Autodesk Inventor part; units mm, degrees
ref_plane "XZ Plane" through (0, 0, 0) normal (0, 1, 0) x (-1, 0, 0)
ref_plane "XY Plane" through (0, 0, 0) normal (0, 0, 1) x (1, 0, 0)
sketch "Sketch1" plane through (0, 0, 0) normal (0, 0, 1) x (1, 0, 0)
  line L0 (125.1975, -635.9781) -> (-63.4844, -635.9781)
  line L1 (-63.4844, -635.9781) -> (-63.4844, -848.7632)
  line L2 (-63.4844, -848.7632) -> (125.1975, -848.7632)
  line L3 (125.1975, -848.7632) -> (125.1975, -635.9781)
  point P0 (0, 0)
extrude "Extrusion1" add sketch "Sketch1" along normal blind 144.4625
sketch "Sketch2" plane through (-63.4844, -848.7632, 0) normal (0, -1, 0) x (1, 0, 0)
  line L0 (188.6819, 144.4625) -> (0, 144.4625)
  line L1 (0, 0) -> (0, 144.4625)
  line L2 (188.6819, 0) -> (188.6819, 144.4625)
  line L3 (0, 17.8487) -> (30.8457, 144.4625)
  line L4 (30.8457, 144.4625) -> (188.6819, 109.8581)
  point P0 (63.4844, 0)
extrude "Extrusion2" cut sketch "Sketch2" against normal through all
sketch "Sketch3" plane through (-63.4844, -848.7632, 17.8487) normal (-0.9715834, 0, 0.2366975) x (0.2366975, 0, 0.9715834)
  line L0 (0, 0) -> (0, 212.7851)
  circle A0 centre (61.7012, 50.3399) radius 23.1304
  line L1 (15.4405, 202.9114) -> (25.6712, 202.9114)
  line L2 (25.6712, 202.9114) -> (25.6712, 176.2225)
  line L3 (25.6712, 176.2225) -> (15.4405, 176.2225)
  line L4 (15.4405, 176.2225) -> (15.4405, 202.9114)
  line L5 (15.4405, 172.4314) -> (25.6712, 172.4314)
  line L6 (25.6712, 172.4314) -> (25.6712, 145.7425)
  line L7 (25.6712, 145.7425) -> (15.4405, 145.7425)
  line L8 (15.4405, 145.7425) -> (15.4405, 172.4314)
  line L9 (15.4405, 141.9514) -> (25.6712, 141.9514)
  line L10 (25.6712, 141.9514) -> (25.6712, 115.2625)
  line L11 (25.6712, 115.2625) -> (15.4405, 115.2625)
  line L12 (15.4405, 115.2625) -> (15.4405, 141.9514)
  point P0 (-2.3149, 848.7632)
  dimension "d6" = 30.48
extrude "Extrusion3" add sketch "Sketch3" along normal blind 12.7
sketch "Sketch4" plane through (-61.219, -798.4232, 80.8026) normal (-0.9715834, 0, 0.2366975) x (0.2366975, 0, 0.9715834)
  circle A0 centre (0, 0) radius 23.1304
  point P0 (-64.0161, 798.4232)
extrude "Extrusion4" add sketch "Sketch4" along normal blind 12.7
sketch "Sketch5" plane through (-63.4844, -848.7632, 17.8487) normal (-0.9715834, 0, 0.2366975) x (0.2366975, 0, 0.9715834)
  circle A0 centre (61.7012, 50.3399) radius 23.1304
  circle A1 centre (61.7012, 50.3399) radius 29.0734 construction
  circle A2 centre (61.7012, 50.3399) radius 43.7714 construction
  line L0 (61.7012, 50.3399) -> (82.0253, 11.5731) construction
  arc A3 (94.4221, 21.2663) -> (38.4943, 67.8529) centre (67.5786, 45.9046) ccw
  line L1 (75.2007, 24.5906) -> (94.4221, 21.2663)
  arc A4 (75.2007, 24.5906) -> (38.4943, 67.8529) centre (61.7012, 50.3399) ccw
  point P0 (-2.3149, 848.7632)
  dimension "d15" = 87.5428
  dimension "d16" = 58.1469
extrude "Extrusion5" cut sketch "Sketch5" along normal mid plane 12.7 contours L1 A4 A3
fillet "Fillet1" radius 130.175 1 edges at (125.1975, -742.3706, 109.8581)
fillet "Fillet2" radius 4.7625 1 edges at (-79.033, -798.4232, 61.3356)
chamfer "Chamfer1" distance 14.2875 angle 45 1 edges at (-32.6387, -742.3706, 144.4625)
ref_plane "Work Plane1" through (119.0625, 0, 0) normal (1, 0, 0) x (0, 1, 0)
sketch "Sketch6" plane through (119.0625, 0, 0) normal (1, 0, 0) x (0, 1, 0)
  circle A0 centre (-684.0193, 29.4352) radius 9.6445
  point P0 (0, 0)
extrude "Extrusion6" add sketch "Sketch6" along normal blind 12.7
properties part number "VoltageSource"
Read the model definition and answer for the solid it produces. Units are mm, in the model's axes. A direction names the side the tool comes from. Give positions to 0.01 mm unless a question says otherwise; leave off trailing zeros. Write each loop counter-clockwise with the first axis right and the second up, starting at its lowest first coordinate (ties: lowest second). Pieces come first, ordered by that corner, then holes. Notation, with made-up numbers: (16, 56) -> (71, 56) arc R20 ccw to (71, 91) -> close; hole circle Ø5 at (9.25, 11.5). An arc over 180 degrees is marked (long way). Answer as a JSON object with one key per item and string values.
1) Straight lines are drawn through the part: probe 1 along X at (y, z) = (-649.5, 49.5); probe 2 along X at (y, z) = (-709.5, 80); probe 3 along Y at (x, z) = (-49.5, 94.5). For each, find the intervals that lie inside material, in ascending order. Write a range as from..to.
Findings below:
{"probe 1": "x = -55.77..117.4", "probe 2": "x = -48.34..101.51", "probe 3": "y = -815.05..-781.8"}
2) Section D-D on x = 62.5 is taken. Write down the section's boundary in (y, z), then the cut area to 3 significant figures.
Findings below:
{"outline": "(-848.76, 0) -> (-635.98, 0) -> (-635.98, 116.45) -> (-848.76, 116.45) -> close", "area": "24,800 mm^2"}
3) A tool of negligible diameter and unlimited length cuts with its end or side. For faces 1 (the flat face through (-65, -706.812, 39)), 2 (the flat face through (-65, -645.852, 39)), 3 (the flat face through (-65.91, -659.38, 34.33)), from which of +Z, -Z, +X, -X, +Y, -Y can it reach the whole face along a straight path? Write none if from no direction.
Findings below:
{"face 1": "+Z, -X", "face 2": "+Z, -X, +Y", "face 3": "-X, +Y, -Y"}
4) For a pull along Y with two mould halves and no side action, classify faces 4 (the flat face through (-63.491, -719.969, 44.272)), 5 (the flat face through (-65, -733.501, 39)), 6 (the flat face through (-65, -676.332, 39)), 7 (the cylindrical face through (127.38, -686.11, 38.85)) as pulls with the +Y half, pulls with the -Y half, needs draft (parallel to the pull), parting line crosses it, or undercut.
Findings below:
{"face 4": "needs draft", "face 5": "pulls with the -Y half", "face 6": "undercut", "face 7": "parting line crosses it"}
5) Section B-B on z = 9 is taken. Write down the section's boundary in (x, y).
Findings below:
{"outline": "(-63.48, -848.76) -> (125.14, -848.76) -> (125.14, -635.98) -> (-63.48, -635.98) -> close"}
6) Flat-ended cylindrical pins translate along their axes: pin 1 Ø4 at (x, z) = (-65.5, 40.5) entering from -Y; pin 2 Ø1 at (y, z) = (-693.5, 117) entering from -X; pin 3 Ø14 at (x, z) = (-68, 39) entering from +Y. Find the tip coordinate at first contact, or state that the pin passes through.
Findings below:
{"pin 1": "stops at y = -733.5", "pin 2": "stops at x = -39.45", "pin 3": "stops at y = -645.85"}
